Source: CAD feature listing. Evaluate the final solid. Frame: model axes, mm. Face numbers are marked on the shaded views. A direction names the side the tool comes from. Round coordinates to 2 decimals unless told otherwise and drop trailing zeros. Loops run counter-clockwise (first coordinate to the right, second up) from the corner with the lowest first, then second, coordinate; pieces in that order, holes last. Notation, with made-up numbers: (14, 59) -> (66, 59) arc R31 ccw to (66, 98) -> close; hole circle Ø3 at (-22.75, -33.5). An arc over 180 degrees is marked (long way). Put each result on its own line as item: value. Start each with the question number.
1. Cut plane A-A (y = 6.5). Return the cut outline in (x, z), then the cut area to 3 significant figures.
2. Contact query for flat-ended pins moving along their axis: pin 1 (3 mm diameter, centred on x = 10.5, z = 18, fed in from -Y); pin 2 (10 mm diameter, centred on y = 30.5, z = 25.5, fed in from +X); pin 3 (0.5 mm diameter, centred on y = 44.5, z = 8.5, fed in from +X). Output: stop coordinate, or through.
3. Cut plane D-D (y = 20.5). Return the cut outline in (x, z), then the cut area to 3 significant figures.
4. Cut plane B-B (z = 14.5). Return the cut outline in (x, y), then the cut area to 3 significant figures.
5. Material intervals for L1, parallel to Z at x = 20, y = 41.5; L2, parallel to Z at x = 6, y = 8; L3, parallel to Z at x = 42, y = 28, sorted ascending.
6. Draft query along X for the marked faces 5, 6, 7 and 8. Return one class per face: pulls with the +X half, pulls with the -X half, needs draft (parallel to the pull), parting line crosses it, or undercut.
7. Cut plane C-C (x = 7). Return the cut outline in (y, z), then the cut area to 3 significant figures.
8. Set-up query: the marked faces 1, 2, 3 and 4. Return all of +Z, -Z, +X, -X, +Y, -Y with unobstructed straight access to the full face (end or side cutting, diameter ignored); none if empty.
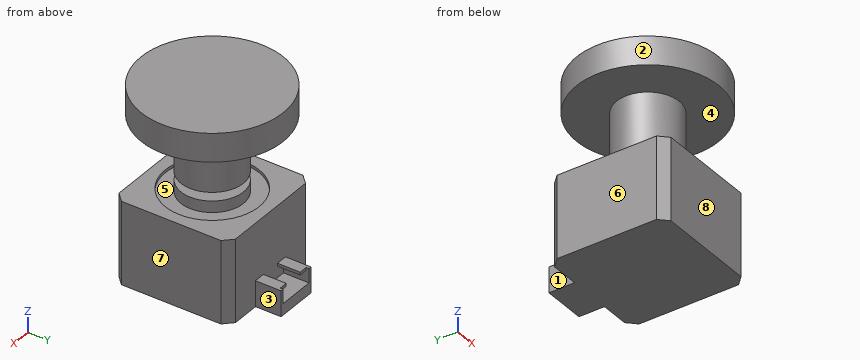
```python
from build123d import *

# Parameters (mm, degrees)
ESQUISSE1_W             = 41
ESQUISSE1_H             = 41
BOSS_EXTRU_1_DEPTH      = 29
ESQUISSE2_R             = 16.5
ESQUISSE2_R_2           = 11
ENL_V_MAT_EXTRU_1_DEPTH = 1
ESQUISSE2_3_R           = 11
ESQUISSE2_3_R_2         = 2.5
BOSS_EXTRU_2_DEPTH      = 3
ESQUISSE2_4_R           = 2.5
BOSS_EXTRU_3_DEPTH      = 6
ESQUISSE7_R             = 11
BOSS_EXTRU_4_DEPTH      = 20
ESQUISSE9_R             = 25
BOSS_EXTRU_5_DEPTH      = 10
CHANFREIN1_SIZE         = 3
ESQUISSE10_W            = 15
ESQUISSE10_H            = 9
ESQUISSE10_W_2          = 13
ESQUISSE10_H_2          = 4
BOSS_EXTRU_6_DEPTH      = 9
ESQUISSE11_W            = 3
ESQUISSE11_H            = 1
ENL_V_MAT_EXTRU_3_DEPTH = 2


with BuildPart() as part:
    # Esquisse1 → Boss.-Extru.1 (new body)
    with BuildSketch(Plane.XY):
        with Locations((20.5, 20.5)):
            Rectangle(ESQUISSE1_W, ESQUISSE1_H)
    extrude(amount=BOSS_EXTRU_1_DEPTH)

    # Esquisse2 → Enl_v. mat.-Extru.1 (cut)
    with BuildSketch(Plane.XY.offset(29)):
        with Locations((20.5, 20.5)):
            Circle(ESQUISSE2_R)
        with Locations((20.5, 20.5)):
            Circle(ESQUISSE2_R_2, mode=Mode.SUBTRACT)
    extrude(amount=-ENL_V_MAT_EXTRU_1_DEPTH, mode=Mode.SUBTRACT)

    # Esquisse2_3 → Boss.-Extru.2 (add)
    with BuildSketch(Plane.XY.offset(29)):
        with Locations((20.5, 20.5)):
            Circle(ESQUISSE2_3_R)
        with Locations((20.5, 20.5)):
            Circle(ESQUISSE2_3_R_2, mode=Mode.SUBTRACT)
    extrude(amount=BOSS_EXTRU_2_DEPTH)

    # Esquisse2_4 → Boss.-Extru.3 (add)
    with BuildSketch(Plane.XY.offset(29)):
        with Locations((20.5, 20.5)):
            Circle(ESQUISSE2_4_R)
    extrude(amount=BOSS_EXTRU_3_DEPTH)

    # Esquisse7 → Boss.-Extru.4 (add)
    with BuildSketch(Plane.XY.offset(35)):
        with Locations((20.5, 20.5)):
            Circle(ESQUISSE7_R)
    extrude(amount=BOSS_EXTRU_4_DEPTH)

    # Esquisse9 → Boss.-Extru.5 (add)
    with BuildSketch(Plane.XY.offset(55)):
        with Locations((20.5, 20.5)):
            Circle(ESQUISSE9_R)
    extrude(amount=BOSS_EXTRU_5_DEPTH)

    # Chanfrein1
    chanfrein1_edges = [part.edges().sort_by_distance(p)[0] for p in [
        (0, 41, 14.5),
        (41, 41, 14.5),
        (41, 0, 14.5),
        (0, 0, 14.5),
    ]]
    chamfer(chanfrein1_edges, length=CHANFREIN1_SIZE)

    # Esquisse10 → Boss.-Extru.6 (add)
    with BuildSketch(Plane(origin=(0, 41, 0), x_dir=(1, 0, 0), z_dir=(0, 1, 0))):
        with Locations((20.5, -4.5)):
            Rectangle(ESQUISSE10_W, ESQUISSE10_H)
        with Locations((20.5, -6)):
            Rectangle(ESQUISSE10_W_2, ESQUISSE10_H_2, mode=Mode.SUBTRACT)
    extrude(amount=BOSS_EXTRU_6_DEPTH)

    # Esquisse11 → Enl_v. mat.-Extru.3 (cut)
    with BuildSketch(Plane.XY.offset(9)):
        with Locations((25.5, 49.5)):
            Rectangle(ESQUISSE11_W, ESQUISSE11_H)
        Polygon((17, 41), (24, 41), (24, 49), (24, 50), (17, 50), (17, 49), align=None)
        with Locations((15.5, 49.5)):
            Rectangle(ESQUISSE11_W, ESQUISSE11_H)
    extrude(amount=-ENL_V_MAT_EXTRU_3_DEPTH, mode=Mode.SUBTRACT)


solid = part.part
```
Solution:
1. outline: (-0.21, 55) -> (41.21, 55) -> (41.21, 65) -> (-0.21, 65) -> close; (0, 0) -> (41, 0) -> (41, 29) -> (29.23, 29) -> (29.23, 28) -> (11.77, 28) -> (11.77, 29) -> (0, 29) -> close
1. area: 1,590 mm^2
2. pin 1: stops at y = 0
2. pin 2: stops at x = 41
2. pin 3: stops at x = 28
3. outline: (-4.5, 55) -> (9.5, 55) -> (9.5, 35) -> (18, 35) -> (18, 32) -> (9.5, 32) -> (9.5, 28) -> (4, 28) -> (4, 29) -> (0, 29) -> (0, 0) -> (41, 0) -> (41, 29) -> (37, 29) -> (37, 28) -> (31.5, 28) -> (31.5, 32) -> (23, 32) -> (23, 35) -> (31.5, 35) -> (31.5, 55) -> (45.5, 55) -> (45.5, 65) -> (-4.5, 65) -> close
3. area: 2,200 mm^2
4. outline: (0, 3) -> (3, 0) -> (38, 0) -> (41, 3) -> (41, 38) -> (38, 41) -> (3, 41) -> (0, 38) -> close
4. area: 1,660 mm^2
5. L1: z = 0 to 4, 55 to 65
5. L2: z = 0 to 29, 55 to 65
5. L3: z = 55 to 65
6. face 5: undercut
6. face 6: pulls with the -X half
6. face 7: pulls with the +X half
6. face 8: needs draft
7. outline: (-0.54, 55) -> (41.54, 55) -> (41.54, 65) -> (-0.54, 65) -> close; (0, 0) -> (41, 0) -> (41, 29) -> (29.99, 29) -> (29.99, 28) -> (11.01, 28) -> (11.01, 29) -> (0, 29) -> close
7. area: 1,590 mm^2
8. face 1: -Z, -X, +Y
8. face 2: +Z
8. face 3: -Z, +X, +Y
8. face 4: none
